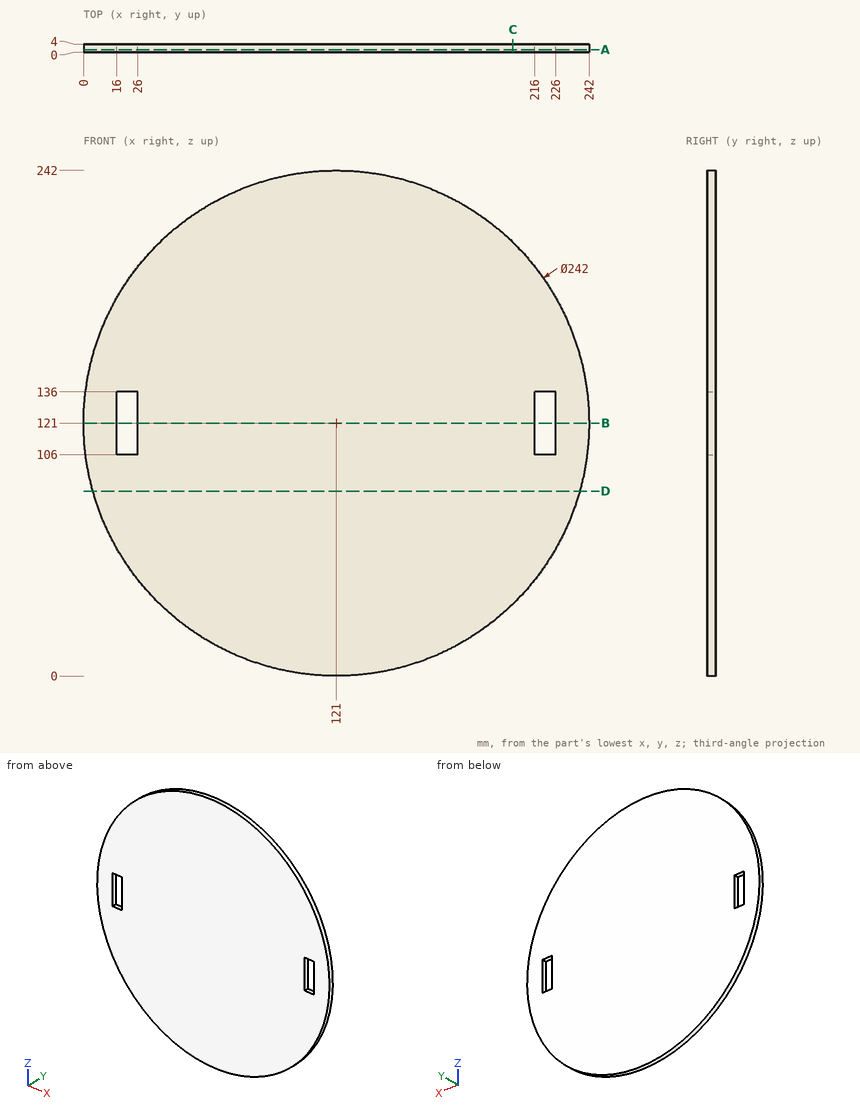
Print and shaded views of the part. All mm, measured from the part's lowest x, y and z. Give positions to 0.01 mm unless a question says otherwise; leave off trailing zeros. Loops run counter-clockwise (first coordinate to the right, second up) from the corner with the lowest first, then second, coordinate; pieces in that order, holes last.
1) Saw through at A-A (y = 1.3). Write the cut outline in (x, z), plus the area to 3 significant figures.
2) Saw through at D-D (z = 88.5). Write the cut outline in (x, y), plus the area to 3 significant figures.
3) Saw through at C-C (x = 205.5). Write the cut outline in (y, z), plus the area to 3 significant figures.
4) Flat gauge pins, fed straight in: pin 1 Ø2 at (x, y) = (104.5, 2) entering from +Z; pin 2 Ø3 at (x, z) = (175, 194.5) entering from -Y; pin 3 Ø2 at (y, z) = (1.5, 126) entering from +X; pin 4 Ø1.5 at (x, y) = (62, 3.5) entering from -Z. Where does each tip first touch, or does it go through?
5) Wall check: line 1 (X direction, y = 2.5, z = 117); line 2 (Z direction, x = 225, y = 1.3); line 3 (X direction, y = 2.1, z = 74.5). Give the ranges that are in metal, low to high.
6) Saw through at B-B (z = 121). Write the cut outline in (x, y), plus the area to 3 significant figures.
Answer block:
1. outline: circle Ø242 at (121, 121); hole (16, 106) - (26, 106) - (26, 136) - (16, 136) - close; hole (216, 106) - (226, 106) - (226, 136) - (216, 136) - close
1. area: 45,400 mm2
2. outline: (4.45, 0) - (237.55, 0) - (237.55, 4) - (4.45, 4) - close
2. area: 932 mm2
3. outline: (0, 34.39) - (4, 34.39) - (4, 207.61) - (0, 207.61) - close
3. area: 693 mm2
4. pin 1: stops at z = 241
4. pin 2: stops at y = 0
4. pin 3: stops at x = 241.93
4. pin 4: stops at z = 14.94
5. line 1: x = 0.07 to 16, 26 to 216, 226 to 241.93
5. line 2: z = 59.15 to 106, 136 to 182.85
5. line 3: x = 9.29 to 232.71
6. outline: (0, 0) - (16, 0) - (16, 4) - (0, 4) - close; (26, 0) - (216, 0) - (216, 4) - (26, 4) - close; (226, 0) - (242, 0) - (242, 4) - (226, 4) - close
6. area: 888 mm2
